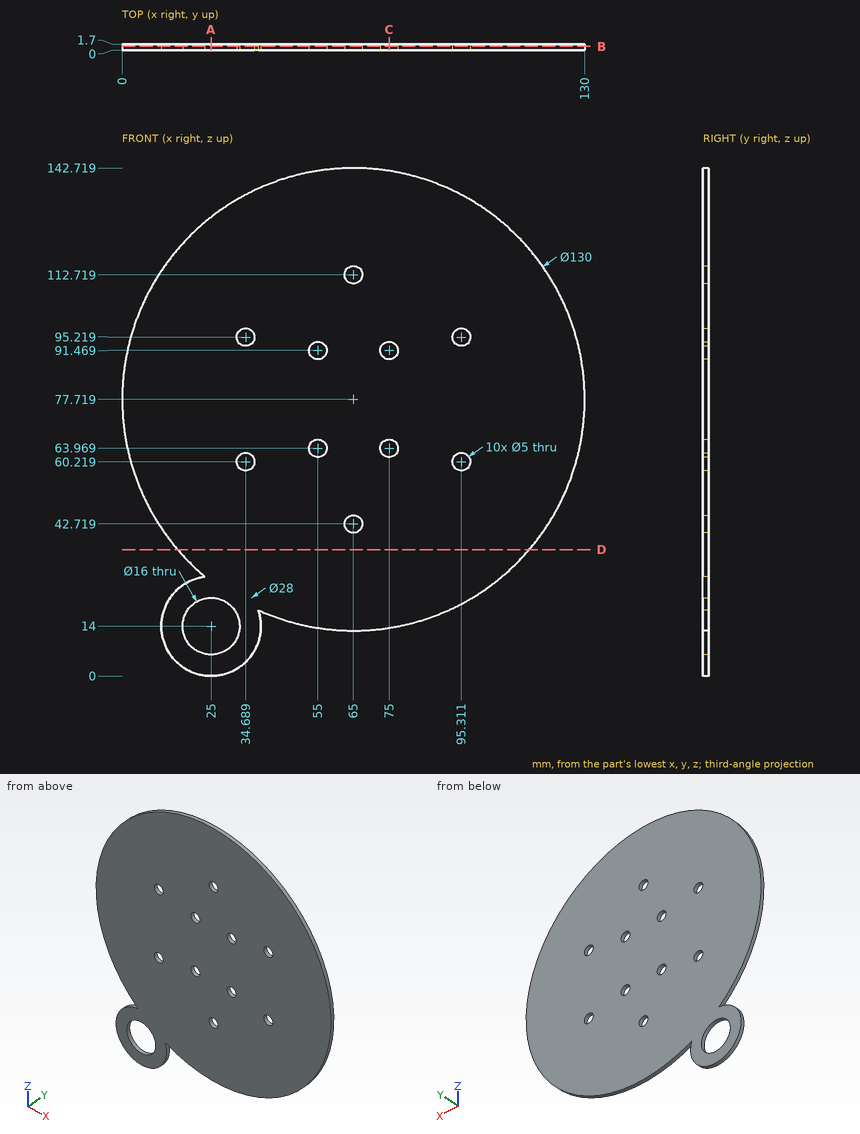
Check sheet for the drawn part. Datum: minimum x, y, z corner. Units: mm. Round coordinates to 2 decimals unless told otherwise and drop trailing zeros. Order: outer loops, then holes, each group sorted by start corner. A loop starts at its lowest first (then second) coordinate and runs counter-clockwise, first axis right, second up. Notation, with made-up numbers: (70.5, -4) -> (125.5, -4) arc R30 cw to (125.5, 24) -> close; hole circle Ø10 at (-22, -40). An arc over 180 degrees is marked (long way). Return JSON: item names as keys, results as strings. Group by question number.
Q1. Section check D-D, the plane z = 35.5. Record the boundary of the cut face in (x, y).
Q2. Gauge pin test, flat end, axial feed: pin 1 (14.5 mm diameter, centred on x = 25, z = 14, fed in from +Y). Record the tip position at first contact, or that the pin passes through.
Q3. Section check C-C, the plane x = 75. Record the boundary of the cut face in (y, z) (1 decimal).
Q4. Section check B-B, the plane y = 1.05. Count the separate pieces of the cut face and the enclosed holes in it, plus the area to 3 significant figures.
Q5. Section check A-A, the plane x = 25. Record the boundary of the cut face in (y, z), plus the area to 3 significant figures.
Q6. Material ranges on probe 1 along Z at (x, y) = (76, 0.55); probe 2 along Z at (x, y) = (74, 1.2) (1 decimal); probe 3 along X at (y, z) = (1.05, 90), recorded low to high. Write a range as from..to.
Numbers:
{
 "1": {"outline": "(15.58, 0) -> (114.42, 0) -> (114.42, 1.7) -> (15.58, 1.7) -> close"},
 "2": {"pin 1": "through"},
 "3": {"outline": "(0, 13.5) -> (1.7, 13.5) -> (1.7, 61.5) -> (0, 61.5) -> close; (0, 66.5) -> (1.7, 66.5) -> (1.7, 89) -> (0, 89) -> close; (0, 94) -> (1.7, 94) -> (1.7, 141.9) -> (0, 141.9) -> close"},
 "4": {"separate pieces": "1", "enclosed holes": "11", "area": "13,400 mm^2"},
 "5": {"outline": "(0, 0) -> (1.7, 0) -> (1.7, 6) -> (0, 6) -> close; (0, 22) -> (1.7, 22) -> (1.7, 128.95) -> (0, 128.95) -> close", "area": "192 mm^2"},
 "6": {"probe 1": "13.66..61.68, 66.26..89.18, 93.76..141.78", "probe 2": "13.3..61.7, 66.3..89.2, 93.8..142.1", "probe 3": "1.17..52.98, 57.02..72.98, 77.02..128.83"}
}
